Geometry: final body of the model. Coordinates: model frame, mm. Face numbers are marked on the shaded views. A direction names the side the tool comes from. Coordinates: 2 decimals unless noted, no trailing zeros. Order: outer loops, then holes, each group sorted by start corner. A loop starts at its lowest first (then second) coordinate and runs counter-clockwise, first axis right, second up. Notation, with made-up numbers: (19, -38) - (39, -38) arc R19 ccw to (39, -10) - close; hole circle Ø5 at (34, -22). An arc over 180 degrees is marked (long way). Use a Markdown table: item, result. Add a question column.
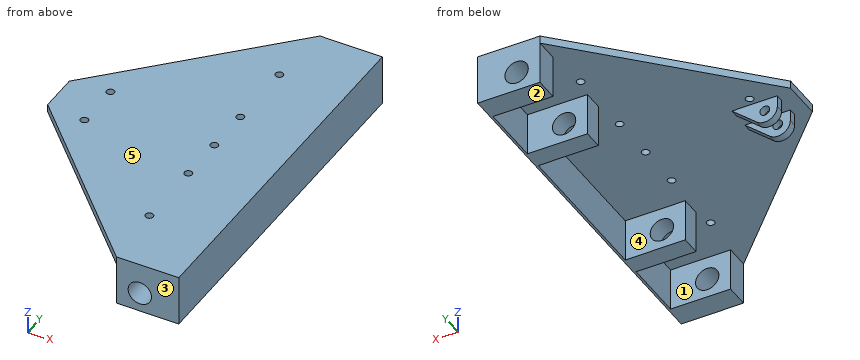
```python
from build123d import *

# Parameters (mm, degrees)
SKETCH2_W               = 80
SKETCH2_H               = 25
BOSS_EXTRUDE1_DEPTH     = 65
BOSS_EXTRUDE1_2_DEPTH   = 65
SKETCH2_W_2             = 70
SKETCH2_H_2             = 10
BOSS_EXTRUDE1_3_DEPTH   = 65
BOSS_EXTRUDE1_4_DEPTH   = 65
SKETCH2_H_3             = 30
BOSS_EXTRUDE1_5_DEPTH   = 65
BOSS_EXTRUDE1_6_DEPTH   = 65
CUT_EXTRUDE1_DEPTH      = 313.209865315
CUT_EXTRUDE1_DEPTH_BACK = 313.209865315
SKETCH3_R               = 15
SKETCH3_R_2             = 6.25
BOSS_EXTRUDE5_DEPTH     = 10
CUT_EXTRUDE2_REACH      = 314.21
SKETCH7_R               = 5
SKETCH8_W               = 65
SKETCH8_H               = 470
BOSS_EXTRUDE6_DEPTH     = 3


with BuildPart() as part:
    # Sketch2 → Boss-Extrude1 (new body)
    with BuildSketch(Plane(origin=(0, 0, 0), x_dir=(1, 0, 0), z_dir=(0, 0, -1))):
        with Locations((155, -112.9)):
            Rectangle(SKETCH2_W, SKETCH2_H)
    extrude(amount=BOSS_EXTRUDE1_DEPTH)


with BuildPart() as body_2:
    # Sketch2 → Boss-Extrude1 2 (new body)
    with BuildSketch(Plane(origin=(0, 0, 0), x_dir=(1, 0, 0), z_dir=(0, 0, -1))):
        with Locations((155, 112.9)):
            Rectangle(SKETCH2_W, SKETCH2_H)
    extrude(amount=BOSS_EXTRUDE1_2_DEPTH)


with BuildPart() as body_3:
    # Sketch2 → Boss-Extrude1 3 (new body)
    with BuildSketch(Plane(origin=(0, 0, 0), x_dir=(1, 0, 0), z_dir=(0, 0, -1))):
        with Locations((-35, 15)):
            Rectangle(SKETCH2_W_2, SKETCH2_H_2)
    extrude(amount=BOSS_EXTRUDE1_3_DEPTH)


with BuildPart() as body_4:
    # Sketch2 → Boss-Extrude1 4 (new body)
    with BuildSketch(Plane(origin=(0, 0, 0), x_dir=(1, 0, 0), z_dir=(0, 0, -1))):
        with Locations((-35, -15)):
            Rectangle(SKETCH2_W_2, SKETCH2_H_2)
    extrude(amount=BOSS_EXTRUDE1_4_DEPTH)


with BuildPart() as body_5:
    # Sketch2 → Boss-Extrude1 5 (new body)
    with BuildSketch(Plane(origin=(0, 0, 0), x_dir=(1, 0, 0), z_dir=(0, 0, -1))):
        with Locations((155, 220)):
            Rectangle(SKETCH2_W, SKETCH2_H_3)
    extrude(amount=BOSS_EXTRUDE1_5_DEPTH)


with BuildPart() as body_6:
    # Sketch2 → Boss-Extrude1 6 (new body)
    with BuildSketch(Plane(origin=(0, 0, 0), x_dir=(1, 0, 0), z_dir=(0, 0, -1))):
        with Locations((155, -220)):
            Rectangle(SKETCH2_W, SKETCH2_H_3)
    extrude(amount=BOSS_EXTRUDE1_6_DEPTH)


with BuildPart() as cut_extrude1_tool:
    # Sketch3 → Cut-Extrude1 (new, two sides: drawn at the far end of the back side and taken through both)
    with BuildSketch(Plane.XZ.offset(-CUT_EXTRUDE1_DEPTH_BACK)):
        with Locations(Location((145, -40, 0), (0, 0, 270))):
            Circle(SKETCH3_R)
        with Locations(Location((-54, -25, 0), (0, 0, 270))):
            Circle(SKETCH3_R_2)
        with BuildLine():
            Line((0, 0), (-43.621584917, -37.17737658))
            ThreePointArc((-43.621584917, -37.17737658), (-60.706167261, -39.526779432), (-70, -25))
            Line((-70, -25), (-75, -25))
            Line((-75, -25), (-75, -70))
            Line((-75, -70), (5, -70))
            Line((5, -70), (5, 0))
            Line((5, 0), (0, 0))
        make_face()
    extrude(amount=CUT_EXTRUDE1_DEPTH + CUT_EXTRUDE1_DEPTH_BACK)


with BuildPart() as part_1:
    add(part.part)

    # Cut-Extrude1: cut by cut_extrude1_tool
    add(cut_extrude1_tool.part, mode=Mode.SUBTRACT)



with BuildPart() as body_2_1:
    add(body_2.part)

    # Cut-Extrude1: cut by cut_extrude1_tool
    add(cut_extrude1_tool.part, mode=Mode.SUBTRACT)


with BuildPart() as body_3_1:
    add(body_3.part)

    # Cut-Extrude1: cut by cut_extrude1_tool
    add(cut_extrude1_tool.part, mode=Mode.SUBTRACT)


with BuildPart() as body_4_1:
    add(body_4.part)

    # Cut-Extrude1: cut by cut_extrude1_tool
    add(cut_extrude1_tool.part, mode=Mode.SUBTRACT)


with BuildPart() as body_5_1:
    add(body_5.part)

    # Cut-Extrude1: cut by cut_extrude1_tool
    add(cut_extrude1_tool.part, mode=Mode.SUBTRACT)


with BuildPart() as body_6_1:
    add(body_6.part)

    # Cut-Extrude1: cut by cut_extrude1_tool
    add(cut_extrude1_tool.part, mode=Mode.SUBTRACT)


with BuildPart() as part_2:
    add(part_1.part)

    add(body_2_1.part)  # Boss-Extrude5 merges body 2

    add(body_3_1.part)  # Boss-Extrude5 merges body 3

    add(body_4_1.part)  # Boss-Extrude5 merges body 4

    add(body_5_1.part)  # Boss-Extrude5 merges body 5

    add(body_6_1.part)  # Boss-Extrude5 merges body 6
    # Sketch6 → Boss-Extrude5 (add)
    with BuildSketch(Plane.XY):
        Polygon((195, 235), (195, -235), (115, -235), (-90, -25), (-90, 25), (115, 235), align=None)
    extrude(amount=-BOSS_EXTRUDE5_DEPTH)

    # Sketch7 → Cut-Extrude2 (cut, up to next)
    with BuildSketch(Plane.XY, mode=Mode.PRIVATE) as cut_extrude2_sk1:
        with Locations((110, 150)):
            Circle(SKETCH7_R)
    cut_extrude2_tool1 = extrude(cut_extrude2_sk1.sketch, amount=-CUT_EXTRUDE2_REACH, mode=Mode.PRIVATE) & part_2.part
    # Sketch7 → Cut-Extrude2 (cut, up to next)
    with BuildSketch(Plane.XY, mode=Mode.PRIVATE) as cut_extrude2_sk2:
        with Locations((110, 60)):
            Circle(SKETCH7_R)
    cut_extrude2_tool2 = extrude(cut_extrude2_sk2.sketch, amount=-CUT_EXTRUDE2_REACH, mode=Mode.PRIVATE) & part_2.part
    # Sketch7 → Cut-Extrude2 (cut, up to next)
    with BuildSketch(Plane.XY, mode=Mode.PRIVATE) as cut_extrude2_sk3:
        with Locations((110, 0)):
            Circle(SKETCH7_R)
    cut_extrude2_tool3 = extrude(cut_extrude2_sk3.sketch, amount=-CUT_EXTRUDE2_REACH, mode=Mode.PRIVATE) & part_2.part
    # Sketch7 → Cut-Extrude2 (cut, up to next)
    with BuildSketch(Plane.XY, mode=Mode.PRIVATE) as cut_extrude2_sk4:
        with Locations((-40, 30)):
            Circle(SKETCH7_R)
    cut_extrude2_tool4 = extrude(cut_extrude2_sk4.sketch, amount=-CUT_EXTRUDE2_REACH, mode=Mode.PRIVATE) & part_2.part
    # Sketch7 → Cut-Extrude2 (cut, up to next)
    with BuildSketch(Plane.XY, mode=Mode.PRIVATE) as cut_extrude2_sk5:
        with Locations(Location((-40, -30, 0), (0, 0, 180))):
            Circle(SKETCH7_R)
    cut_extrude2_tool5 = extrude(cut_extrude2_sk5.sketch, amount=-CUT_EXTRUDE2_REACH, mode=Mode.PRIVATE) & part_2.part
    # Sketch7 → Cut-Extrude2 (cut, up to next)
    with BuildSketch(Plane.XY, mode=Mode.PRIVATE) as cut_extrude2_sk6:
        with Locations(Location((110, -60, 0), (0, 0, 180))):
            Circle(SKETCH7_R)
    cut_extrude2_tool6 = extrude(cut_extrude2_sk6.sketch, amount=-CUT_EXTRUDE2_REACH, mode=Mode.PRIVATE) & part_2.part
    # Sketch7 → Cut-Extrude2 (cut, up to next)
    with BuildSketch(Plane.XY, mode=Mode.PRIVATE) as cut_extrude2_sk7:
        with Locations(Location((110, -150, 0), (0, 0, 180))):
            Circle(SKETCH7_R)
    cut_extrude2_tool7 = extrude(cut_extrude2_sk7.sketch, amount=-CUT_EXTRUDE2_REACH, mode=Mode.PRIVATE) & part_2.part
    add(cut_extrude2_tool1.solids().sort_by_distance((110, 150, 0))[0], mode=Mode.SUBTRACT)
    add(cut_extrude2_tool2.solids().sort_by_distance((110, 60, 0))[0], mode=Mode.SUBTRACT)
    add(cut_extrude2_tool3.solids().sort_by_distance((110, 0, 0))[0], mode=Mode.SUBTRACT)
    add(cut_extrude2_tool4.solids().sort_by_distance((-40, 30, 0))[0], mode=Mode.SUBTRACT)
    add(cut_extrude2_tool5.solids().sort_by_distance((-40, -30, 0))[0], mode=Mode.SUBTRACT)
    add(cut_extrude2_tool6.solids().sort_by_distance((110, -60, 0))[0], mode=Mode.SUBTRACT)
    add(cut_extrude2_tool7.solids().sort_by_distance((110, -150, 0))[0], mode=Mode.SUBTRACT)

    # Sketch8 → Boss-Extrude6 (add)
    with BuildSketch(Plane(origin=(195, 0, 0), x_dir=(0, 0, -1), z_dir=(1, 0, 0))):
        with Locations((32.5, 0)):
            Rectangle(SKETCH8_W, SKETCH8_H)
    extrude(amount=-BOSS_EXTRUDE6_DEPTH)


solid = part_2.part
```
1) Draft query along Y for the marked faces 1, 2 and 3. Return one class per face: released by +Y, released by -Y, zero draft, split by the parting line, or undercut.
2) Section query B-B (x = 110). Return the cut outline in (y, z).
3) Section query A-A (y = 60). Return the cut outline in (x, z).
4) First-contact query: pin 1 (6 mm diameter, centred on x = 110, y = -150, fed in from -Z); pin 2 (8 mm diameter, centred on y = -159.5, z = -46.5, fed in from -X); pin 3 (16 mm diameter, centred on x = -54, z = -25, fed in from -Y); pin 4 (11.5 mm diameter, centred on x = 110, y = 0, fed in from -Z). Flat tips, straight axial feed; report the tip coordinate or a pass-through.
5) Line query: line 1 (Y direction, x = 154, z = -56); line 2 (X direction, y = 12, z = -25); line 3 (Y direction, x = -43.5, z = -7). Output: solid intervals per line, ascending. Write a range as from..to.
6) Section query C-C (y = 114.5). Return the cut outline in (x, z), and give its area (3 significant figures).
7) Access query for the marked faces 4 and 5. Directions: +Z, -Z, +X, -X, +Y, -Y. A direction counts if a zero-diameter tool reaches every point of the face in a straight line with its end or side. Return the directions, or none.
8) Section query D-D (y = -159.5). Return the cut outline in (x, z), and give its area (3 significant figures).
From the geometry:
| question | item | result |
|---|---|---|
| 1 | face 1 | undercut |
| 1 | face 2 | zero draft |
| 1 | face 3 | released by -Y |
| 2 | outline | (-229.88, -10) - (-155, -10) - (-155, 0) - (-229.88, 0) - close; (-145, -10) - (-65, -10) - (-65, 0) - (-145, 0) - close; (-55, -10) - (-5, -10) - (-5, 0) - (-55, 0) - close; (5, -10) - (55, -10) - (55, 0) - (5, 0) - close; (65, -10) - (145, -10) - (145, 0) - (65, 0) - close; (155, -10) - (229.88, -10) - (229.88, 0) - (155, 0) - close |
| 3 | outline | (-55.83, -10) - (105, -10) - (105, 0) - (-55.83, 0) - close; (115, -10) - (192, -10) - (192, -65) - (195, -65) - (195, 0) - (115, 0) - close |
| 4 | pin 1 | passes through |
| 4 | pin 2 | stops at x = 192 |
| 4 | pin 3 | stops at y = -20 |
| 4 | pin 4 | stops at z = -10 |
| 5 | line 1 | y = -235..-205, -125.4..-100.4, 100.4..125.4, 205..235 |
| 5 | line 2 | x = -70..-60.25, -47.75..-29.33, 192..195 |
| 5 | line 3 | y = -72.63..-33.57, -26.43..26.43, 33.57..72.63 |
| 6 | outline | (-2.63, -10) - (115, -10) - (115, -65) - (195, -65) - (195, 0) - (-2.63, 0) - close; hole circle Ø30 at (145, -40) |
| 6 | area | 5,670 mm^2 |
| 7 | face 4 | -Z, -X |
| 7 | face 5 | +Z, +X, -X, +Y, -Y |
| 8 | outline | (41.3, -10) - (192, -10) - (192, -65) - (195, -65) - (195, 0) - (41.3, 0) - close |
| 8 | area | 1,700 mm^2 |
